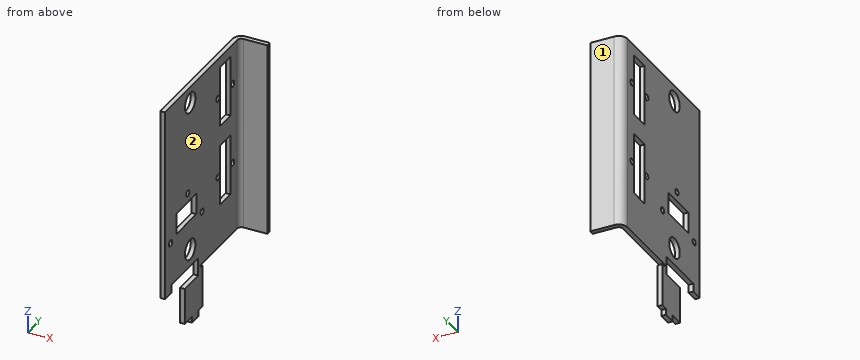
from build123d import *

# Parameters (mm, degrees)
BASE_FLANGE1_DEPTH      = 94.85
BASE_FLANGE1_DEPTH_BACK = 25.65
SKETCH7_R               = 1.5
SKETCH7_R_2             = 5
SKETCH7_W               = 10.4
SKETCH7_H               = 19
SKETCH7_W_2             = 30
SKETCH7_H_2             = 10
CUT_EXTRUDE2_DEPTH      = 121.75397509


# Sheet-metal steps are written as plain solids
with BuildPart() as part:
    # Sketch2 → Base-Flange1 (new, two sides: drawn at the far end of the back side and taken through both)
    with BuildSketch(Plane.XY.offset(-BASE_FLANGE1_DEPTH_BACK)):
        with BuildLine():
            Line((0, 0), (0, 68.7))
            ThreePointArc((0, 68.7), (1.259440841, 71.740559159), (4.3, 73))
            Line((4.3, 73), (16, 73))
            Line((16, 73), (16, 70.7))
            Line((16, 70.7), (4.3, 70.7))
            ThreePointArc((4.3, 70.7), (2.885786438, 70.114213562), (2.3, 68.7))
            Line((2.3, 68.7), (2.3, 0))
            Line((2.3, 0), (0, 0))
        make_face()
    extrude(amount=BASE_FLANGE1_DEPTH + BASE_FLANGE1_DEPTH_BACK)

    # Sketch7 → Cut-Extrude2 (cut, through all)
    with BuildSketch(Plane.ZY):
        with Locations((34.85, 64.4)):
            Circle(SKETCH7_R)
        with Locations((34.85, 50.4)):
            Circle(SKETCH7_R)
        with Locations((74.85, 64.4)):
            Circle(SKETCH7_R)
        with Locations((74.85, 50.4)):
            Circle(SKETCH7_R)
        with Locations((25.55, 35.3)):
            Circle(SKETCH7_R)
        with Locations((25.55, 5.3)):
            Circle(SKETCH7_R)
        with Locations((42.15, 21.7)):
            Circle(SKETCH7_R)
        with Locations((87, 24)):
            Circle(SKETCH7_R_2)
        with Locations((12.5, 24)):
            Circle(SKETCH7_R_2)
        with Locations((32.45, 20.3)):
            Rectangle(SKETCH7_W, SKETCH7_H)
        with Locations((74.85, 57.4)):
            Rectangle(SKETCH7_W_2, SKETCH7_H_2)
        with Locations((34.85, 57.4)):
            Rectangle(SKETCH7_W_2, SKETCH7_H_2)
        Polygon((-0.85, 33.637171027), (-1.85, 33.637171027), (-1.85, 35.637171027), (-22.65, 35.637171027), (-22.65, 32.037171027), (-25.65, 32.037171027), (-25.65, 73), (-0.85, 73), align=None)
        Polygon((-22.65, 25.737171027), (-22.65, 18.837171027), (-4.85, 18.837171027), (-4.85, 31.5), (4, 31.5), (4, 6.1), (0, 6.1), (0, 0), (-25.65, 0), (-25.65, 25.737171027), align=None)
    extrude(amount=-CUT_EXTRUDE2_DEPTH, mode=Mode.SUBTRACT)


solid = part.part
Source: CAD feature listing. Evaluate the final solid. Frame: model axes, mm. Face numbers are marked on the shaded views. A direction names the side the tool comes from. Round coordinates to 2 decimals unless told otherwise and drop trailing zeros. Write each loop counter-clockwise with the first axis right and the second up, starting at its lowest first coordinate (ties: lowest second). Pieces come first, ordered by that corner, then holes. Notation, with made-up numbers: M 6,-5 L 44,-5 A21 ccw 44,4 Z; hole C 78,61 d6. An arc over 180 degrees is marked long. One line per item, written item: value. Start each with the question number.
Item 1: Ray query, L1, parallel to Y at x = 1.2, z = 34.85; L2, parallel to Y at x = 1.45, z = 34.85; L3, parallel to Y at x = 0.9, z = 74.85. Return the intervals inside material, ascending. Write a range as from..to.
Item 2: Pin query (flat end, axial travel): pin 1 (0.7 mm diameter, centred on x = 0.5, z = -10, fed in from -Y); pin 2 (1 mm diameter, centred on y = 39, z = 1, fed in from +X); pin 3 (8 mm diameter, centred on x = 13.5, z = 82.5, fed in from -Y). Return the tip coordinate at first contact, or that it passes through.
Item 3: Section query C-C (y = 12). Return the cut outline in (x, z).
Item 4: Section query D-D (z = 87). Return the cut outline in (x, y).
Item 5: Section query A-A (y = 50.4). Return the cut outline in (x, z).
Item 6: Section query B-B (z = 42.15). Return the cut outline in (x, y).
Item 7: Set-up query: the marked faces 1 and 2. Return all of +Z, -Z, +X, -X, +Y, -Y with unobstructed straight access to the full face (end or side cutting, diameter ignored); none if empty.
Result set:
1. L1: y = 0..10.8, 29.8..48.9, 51.9..52.4, 62.4..62.9, 65.9..71.68
1. L2: y = 0..10.8, 29.8..48.9, 51.9..52.4, 62.4..62.9, 65.9..71.92
1. L3: y = 0..48.9, 51.9..52.4, 62.4..62.9, 65.9..71.33
2. pin 1: stops at y = 18.84
2. pin 2: stops at x = 2.3
2. pin 3: stops at y = 70.7
3. outline: M 0,4 L 2.3,4 L 2.3,27.25 L 0,27.25 Z; M 0,37.65 L 2.3,37.65 L 2.3,94.85 L 0,94.85 Z
4. outline: M 0,0 L 2.3,0 L 2.3,19 L 0,19 Z; M 0,29 L 2.3,29 L 2.3,52.4 L 0,52.4 Z; M 0,62.4 L 2.3,62.4 L 2.3,68.7 A2 cw 4.3,70.7 L 16,70.7 L 16,73 L 4.3,73 A4.3 ccw 0,68.7 Z
5. outline: M 0,-0.85 L 2.3,-0.85 L 2.3,33.35 L 0,33.35 Z; M 0,36.35 L 2.3,36.35 L 2.3,73.35 L 0,73.35 Z; M 0,76.35 L 2.3,76.35 L 2.3,94.85 L 0,94.85 Z
6. outline: M 0,0 L 2.3,0 L 2.3,20.2 L 0,20.2 Z; M 0,23.2 L 2.3,23.2 L 2.3,52.4 L 0,52.4 Z; M 0,62.4 L 2.3,62.4 L 2.3,68.7 A2 cw 4.3,70.7 L 16,70.7 L 16,73 L 4.3,73 A4.3 ccw 0,68.7 Z
7. face 1: +Z, -Z, +X, -X, +Y
7. face 2: +Z, -Z, +X, -Y
